Model file for the job. Use its own axes, mm. A direction names the side the tool comes from. Give positions to 0.01 mm unless a question says otherwise; leave off trailing zeros. Order: outer loops, then holes, each group sorted by start corner. A loop starts at its lowest first (then second) coordinate and runs counter-clockwise, first axis right, second up. Notation, with made-up numbers: (71, -24.5) -> (97, -24.5) arc R27 cw to (97, 5.5) -> close; hole circle Ø2 at (76, 37). An arc over 180 degrees is marked (long way). Answer in a Markdown table with one row per item. Add a question column.
from build123d import *

# Parameters (mm, degrees)
SKETCH_W        = 70.3
SKETCH_H        = 51
PAD_DEPTH       = 50.65
SKETCH001_W     = 44.3
SKETCH001_H     = 47.65
SKETCH001_W_2   = 10
POCKET_DEPTH    = 51.001
SKETCH002_R     = 3
SKETCH002_R_2   = 2
SKETCH002_W     = 15
SKETCH002_H     = 15
POCKET001_DEPTH = 50.651


with BuildPart() as part:
    # Sketch → Pad (new body)
    with BuildSketch(Plane.XY):
        with Locations((35.15, 25.5)):
            Rectangle(SKETCH_W, SKETCH_H)
    extrude(amount=PAD_DEPTH)

    # Sketch001 → Pocket (cut, through all)
    with BuildSketch(Plane.XZ):
        with Locations((35.15, 23.825)):
            Rectangle(SKETCH001_W, SKETCH001_H)
        with Locations((5, 26.825)):
            Rectangle(SKETCH001_W_2, SKETCH001_H)
        with Locations((65.3, 26.825)):
            Rectangle(SKETCH001_W_2, SKETCH001_H)
    extrude(amount=-POCKET_DEPTH, mode=Mode.SUBTRACT)

    # Sketch002 → Pocket001 (cut, through all)
    with BuildSketch(Plane.XY.offset(50.65)):
        with Locations((20, 41)):
            Circle(SKETCH002_R)
        with Locations((50.3, 41)):
            Circle(SKETCH002_R)
        with Locations((20, 10)):
            Circle(SKETCH002_R)
        with Locations((50.3, 10)):
            Circle(SKETCH002_R)
        with Locations((4, 40.8)):
            Circle(SKETCH002_R_2)
        with Locations((4, 30.6)):
            Circle(SKETCH002_R_2)
        with Locations((4, 20.4)):
            Circle(SKETCH002_R_2)
        with Locations((4, 10.2)):
            Circle(SKETCH002_R_2)
        with Locations((66.3, 40.8)):
            Circle(SKETCH002_R_2)
        with Locations((66.3, 30.6)):
            Circle(SKETCH002_R_2)
        with Locations((66.3, 20.4)):
            Circle(SKETCH002_R_2)
        with Locations((66.3, 10.2)):
            Circle(SKETCH002_R_2)
        with Locations((35.15, 43.5)):
            Rectangle(SKETCH002_W, SKETCH002_H)
    extrude(amount=-POCKET001_DEPTH, mode=Mode.SUBTRACT)


solid = part.part
Item 1: Pin check, flat tips, straight feed: pin 1 Ø24 at (y, z) = (22.5, 24.5) entering from -X; pin 2 Ø7 at (x, y) = (20, 41) entering from -Z; pin 3 Ø6.5 at (x, y) = (4, 30.6) entering from +Z. Stop position of each tip, or through.
Item 2: Wall check: line 1 (Y direction, x = 4, z = 1); line 2 (Y direction, x = 20, z = 49); line 3 (X direction, y = 16.5, z = 32). Give the ranges that are in metal, low to high.
Item 3: Saw through at B-B on y = 30.6. List the corners of the cut face in (x, z), plus the area to 3 significant figures.
Item 4: Saw through at D-D on y = 45. List the corners of the cut face in (x, z).
Item 5: Which spindle directions (+Z, -Z, +X, -X, +Y, -Y) get a long thin tool onto all of the face, cutting with end or side? Do faces 1 (the cylindrical face through (2.4, 29.4, 1.5)), 2 (the flat face through (42.65, 43, 49)), 3 (the flat face through (57.3, 25, 23)). Say none if no direction does.
Item 6: Saw through at C-C on x = 48.5. List the corners of the cut face in (y, z).
Item 7: Saw through at A-A on z = 6. List the corners of the cut face in (x, y).
Evaluation:
| question | item | result |
|---|---|---|
| 1 | pin 1 | stops at x = 10 |
| 1 | pin 2 | stops at z = 47.65 |
| 1 | pin 3 | stops at z = 3 |
| 2 | line 1 | y = 0 to 8.2, 12.2 to 18.4, 22.4 to 28.6, 32.6 to 38.8, 42.8 to 51 |
| 2 | line 2 | y = 0 to 7, 13 to 38, 44 to 51 |
| 2 | line 3 | x = 10 to 13, 57.3 to 60.3 |
| 3 | outline | (0, 0) -> (2, 0) -> (2, 3) -> (0, 3) -> close; (6, 0) -> (13, 0) -> (13, 47.65) -> (57.3, 47.65) -> (57.3, 0) -> (64.3, 0) -> (64.3, 3) -> (60.3, 3) -> (60.3, 50.65) -> (10, 50.65) -> (10, 3) -> (6, 3) -> close; (68.3, 0) -> (70.3, 0) -> (70.3, 3) -> (68.3, 3) -> close |
| 3 | area | 473 mm2 |
| 4 | outline | (0, 0) -> (13, 0) -> (13, 47.65) -> (27.65, 47.65) -> (27.65, 50.65) -> (10, 50.65) -> (10, 3) -> (0, 3) -> close; (42.65, 47.65) -> (57.3, 47.65) -> (57.3, 0) -> (70.3, 0) -> (70.3, 3) -> (60.3, 3) -> (60.3, 50.65) -> (42.65, 50.65) -> close |
| 5 | face 1 | +Z, -Z |
| 5 | face 2 | +Z, -Z, +Y |
| 5 | face 3 | -Z, +Y, -Y |
| 6 | outline | (0, 47.65) -> (7.6, 47.65) -> (7.6, 50.65) -> (0, 50.65) -> close; (12.4, 47.65) -> (38.6, 47.65) -> (38.6, 50.65) -> (12.4, 50.65) -> close; (43.4, 47.65) -> (51, 47.65) -> (51, 50.65) -> (43.4, 50.65) -> close |
| 7 | outline | (10, 0) -> (13, 0) -> (13, 51) -> (10, 51) -> close; (57.3, 0) -> (60.3, 0) -> (60.3, 51) -> (57.3, 51) -> close |
